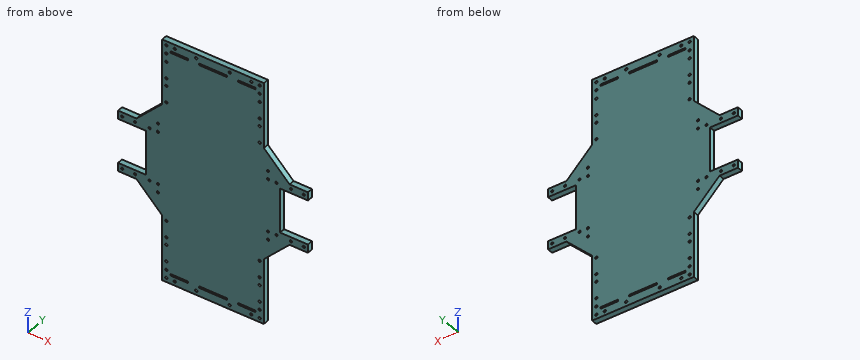
```python
from build123d import *

# Parameters (mm, degrees)
BOSS_EXTRUDE1_DEPTH = 10
SKETCH2_R           = 2
SKETCH2_W           = 50
SKETCH2_H           = 80
CUT_EXTRUDE1_DEPTH  = 278.418456488
SKETCH3_R           = 2.1
SKETCH3_W           = 50
SKETCH3_H           = 3
SKETCH3_W_2         = 31
CUT_EXTRUDE2_DEPTH  = 278.418456488


with BuildPart() as part:
    # Sketch1 → Boss-Extrude1 (new body)
    with BuildSketch(Plane(origin=(0, 0, 0), x_dir=(1, 0, 0), z_dir=(0, 1, 0))):
        Polygon((-91, -219), (91, -219), (91, -101), (137, -55), (170, -55), (170, 55), (137, 55), (91, 101), (91, 219), (-91, 219), (-91, 101), (-137, 55), (-170, 55), (-170, -55), (-137, -55), (-91, -101), align=None)
    extrude(amount=BOSS_EXTRUDE1_DEPTH)

    # Sketch2 → Cut-Extrude1 (cut, through all)
    with BuildSketch(Plane(origin=(0, 10, 0), x_dir=(1, 0, 0), z_dir=(0, 1, 0))):
        with Locations(Location((-162.5, 47.5, 0), (0, 0, 270))):
            Circle(SKETCH2_R)
        with Locations(Location((-139.5, 47.5, 0), (0, 0, 270))):
            Circle(SKETCH2_R)
        with Locations(Location((-139.5, -47.5, 0), (0, 0, 90))):
            Circle(SKETCH2_R)
        with Locations(Location((-162.5, -47.5, 0), (0, 0, 90))):
            Circle(SKETCH2_R)
        with Locations(Location((-113.5, 47.5, 0), (0, 0, 270))):
            Circle(SKETCH2_R)
        with Locations(Location((-98.5, 47.5, 0), (0, 0, 270))):
            Circle(SKETCH2_R)
        with Locations(Location((-98.5, 62.5, 0), (0, 0, 270))):
            Circle(SKETCH2_R)
        with Locations(Location((-98.5, -62.5, 0), (0, 0, 90))):
            Circle(SKETCH2_R)
        with Locations(Location((-98.5, -47.5, 0), (0, 0, 90))):
            Circle(SKETCH2_R)
        with Locations(Location((-113.5, -47.5, 0), (0, 0, 90))):
            Circle(SKETCH2_R)
        with Locations(Location((113.5, -47.5, 0), (0, 0, 270))):
            Circle(SKETCH2_R)
        with Locations(Location((98.5, -47.5, 0), (0, 0, 270))):
            Circle(SKETCH2_R)
        with Locations(Location((98.5, -62.5, 0), (0, 0, 270))):
            Circle(SKETCH2_R)
        with Locations(Location((98.5, 62.5, 0), (0, 0, 90))):
            Circle(SKETCH2_R)
        with Locations(Location((98.5, 47.5, 0), (0, 0, 90))):
            Circle(SKETCH2_R)
        with Locations(Location((113.5, 47.5, 0), (0, 0, 90))):
            Circle(SKETCH2_R)
        with Locations(Location((162.5, -47.5, 0), (0, 0, 270))):
            Circle(SKETCH2_R)
        with Locations(Location((139.5, -47.5, 0), (0, 0, 270))):
            Circle(SKETCH2_R)
        with Locations(Location((139.5, 47.5, 0), (0, 0, 90))):
            Circle(SKETCH2_R)
        with Locations(Location((162.5, 47.5, 0), (0, 0, 90))):
            Circle(SKETCH2_R)
        with Locations((-145, 0)):
            Rectangle(SKETCH2_W, SKETCH2_H)
        with Locations((145, 0)):
            Rectangle(SKETCH2_W, SKETCH2_H)
    extrude(amount=-CUT_EXTRUDE1_DEPTH, mode=Mode.SUBTRACT)

    # Sketch3 → Cut-Extrude2 (cut, through all)
    with BuildSketch(Plane(origin=(0, 10, 0), x_dir=(1, 0, 0), z_dir=(0, 1, 0))):
        with Locations(Location((-30, 211.5, 0), (0, 0, 270))):
            Circle(SKETCH3_R)
        with Locations(Location((30, 211.5, 0), (0, 0, 270))):
            Circle(SKETCH3_R)
        with Locations(Location((68.5, 211.5, 0), (0, 0, 270))):
            Circle(SKETCH3_R)
        with Locations(Location((83.5, 211.5, 0), (0, 0, 270))):
            Circle(SKETCH3_R)
        with Locations(Location((83.5, 196.5, 0), (0, 0, 270))):
            Circle(SKETCH3_R)
        with Locations(Location((83.5, 181.5, 0), (0, 0, 270))):
            Circle(SKETCH3_R)
        with Locations(Location((83.5, 151.5, 0), (0, 0, 270))):
            Circle(SKETCH3_R)
        with Locations(Location((83.5, 137.5, 0), (0, 0, 270))):
            Circle(SKETCH3_R)
        with Locations(Location((83.5, 107.5, 0), (0, 0, 270))):
            Circle(SKETCH3_R)
        with Locations(Location((-83.5, 107.5, 0), (0, 0, 90))):
            Circle(SKETCH3_R)
        with Locations(Location((-83.5, 137.5, 0), (0, 0, 90))):
            Circle(SKETCH3_R)
        with Locations(Location((-83.5, 151.5, 0), (0, 0, 90))):
            Circle(SKETCH3_R)
        with Locations(Location((-83.5, 181.5, 0), (0, 0, 90))):
            Circle(SKETCH3_R)
        with Locations(Location((-83.5, 196.5, 0), (0, 0, 90))):
            Circle(SKETCH3_R)
        with Locations(Location((-83.5, 211.5, 0), (0, 0, 90))):
            Circle(SKETCH3_R)
        with Locations(Location((-68.5, 211.5, 0), (0, 0, 90))):
            Circle(SKETCH3_R)
        with Locations(Location((-68.5, -211.5, 0), (0, 0, 270))):
            Circle(SKETCH3_R)
        with Locations(Location((-83.5, -211.5, 0), (0, 0, 270))):
            Circle(SKETCH3_R)
        with Locations(Location((-83.5, -196.5, 0), (0, 0, 270))):
            Circle(SKETCH3_R)
        with Locations(Location((-83.5, -181.5, 0), (0, 0, 270))):
            Circle(SKETCH3_R)
        with Locations(Location((-83.5, -151.5, 0), (0, 0, 270))):
            Circle(SKETCH3_R)
        with Locations(Location((-83.5, -137.5, 0), (0, 0, 270))):
            Circle(SKETCH3_R)
        with Locations(Location((-83.5, -107.5, 0), (0, 0, 270))):
            Circle(SKETCH3_R)
        with Locations(Location((83.5, -107.5, 0), (0, 0, 90))):
            Circle(SKETCH3_R)
        with Locations(Location((83.5, -137.5, 0), (0, 0, 90))):
            Circle(SKETCH3_R)
        with Locations(Location((83.5, -151.5, 0), (0, 0, 90))):
            Circle(SKETCH3_R)
        with Locations(Location((83.5, -181.5, 0), (0, 0, 90))):
            Circle(SKETCH3_R)
        with Locations(Location((83.5, -196.5, 0), (0, 0, 90))):
            Circle(SKETCH3_R)
        with Locations(Location((83.5, -211.5, 0), (0, 0, 90))):
            Circle(SKETCH3_R)
        with Locations(Location((68.5, -211.5, 0), (0, 0, 90))):
            Circle(SKETCH3_R)
        with Locations(Location((30, -211.5, 0), (0, 0, 90))):
            Circle(SKETCH3_R)
        with Locations(Location((-30, -211.5, 0), (0, 0, 90))):
            Circle(SKETCH3_R)
        with Locations((0, 202.5)):
            Rectangle(SKETCH3_W, SKETCH3_H)
        with Locations((60.5, 202.5)):
            Rectangle(SKETCH3_W_2, SKETCH3_H)
        with Locations((-60.5, 202.5)):
            Rectangle(SKETCH3_W_2, SKETCH3_H)
        with Locations((-60.5, -202.5)):
            Rectangle(SKETCH3_W_2, SKETCH3_H)
        with Locations((60.5, -202.5)):
            Rectangle(SKETCH3_W_2, SKETCH3_H)
        with Locations((0, -202.5)):
            Rectangle(SKETCH3_W, SKETCH3_H)
    extrude(amount=-CUT_EXTRUDE2_DEPTH, mode=Mode.SUBTRACT)


solid = part.part
```
Check sheet for the modelled part. Datum: model origin and axes. Units: mm. Give positions to 0.01 mm unless a question says otherwise; leave off trailing zeros. Loops run counter-clockwise (first coordinate to the right, second up) from the corner with the lowest first, then second, coordinate; pieces in that order, holes last. Notation, with made-up numbers: M 81.25,28.5 L 100.25,28.5 A29 cw 100.25,53.5 Z; hole C 9.5,71 d6. An arc over 180 degrees is marked long. Answer in a Markdown table with one row per item.
1) Thickness scan on line 1 (Z direction, x = 48.5, y = 1.5); line 2 (Z direction, x = -162.5, y = 5.5); line 3 (X direction, y = 6.5, z = 151.5). Record the ranges inside material, lowest first.
Solutions:
| item | result |
|---|---|
| line 1 | z = -219 to -204, -201 to 201, 204 to 219 |
| line 2 | z = -55 to -49.5, -45.5 to -40, 40 to 45.5, 49.5 to 55 |
| line 3 | x = -91 to -85.6, -81.4 to 81.4, 85.6 to 91 |
2) Depth check by flat-ended pin: pin 1 (4 mm diameter, centred on x = -110, y = 2, fed in from -Z); pin 2 (3 mm diameter, centred on y = 4, z = 119, fed in from -X); pin 3 (6.5 mm diameter, centred on x = 83.5, z = -151.5, fed in from -Y); pin 4 (6 mm diameter, centred on x = -112.5, y = 6.5, fed in from -Z). Enter the tip coordinate at first touch or a pass-through.
Solutions:
| item | result |
|---|---|
| pin 1 | stops at z = -84 |
| pin 2 | stops at x = -91 |
| pin 3 | stops at y = 0 |
| pin 4 | stops at z = -82.5 |
3) Cross-section at A-A (z = 28). Enter the section's corners in (x, y).
Solutions:
| item | result |
|---|---|
| outline | M -120,0 L 120,0 L 120,10 L -120,10 Z |
4) Cross-section at B-B (y = 2). Count the separate pieces of the cut face and the enclosed holes in it, plus the area to 3 significant figures.
Solutions:
| item | result |
|---|---|
| separate pieces | 1 |
| enclosed holes | 58 |
| area | 92,000 mm^2 |
